Source: CAD feature listing. Evaluate the final solid. Frame: model axes, mm. A direction names the side the tool comes from. Give positions to 0.01 mm unless a question says otherwise; leave off trailing zeros. Order: outer loops, then holes, each group sorted by start corner. A loop starts at its lowest first (then second) coordinate and runs counter-clockwise, first axis right, second up.
```python
from build123d import *

# Parameters (mm, degrees)
F1_DEPTH  = 530
F0_R      = 50
F0_R_2    = 45
F2_DEPTH  = 9
F3_R      = 150.0861563529
F3_R_2    = 146
F3_R_3    = 144
F3_R_4    = 138
F4_DEPTH  = 15
F5_DEPTH  = 15
F7_R      = 141.9845884843
F8_DEPTH  = 15
F9_W      = 99.9695800245
F9_H      = 293.9526891708
F9_H_2    = 15
F10_DEPTH = 15
F11_W     = 99.9695800245
F11_H     = 308.8312447071
F12_DEPTH = 15
F14_DEPTH = 309
F15_DEPTH = 15
F16_DEPTH = 5
F17_R     = 2


with BuildPart() as f1:
    # F0 (on Front) → F1 (new body)
    with BuildSketch(Plane.XZ):
        with BuildLine():
            Line((50, 135.0407345952), (50, 137.1714255959))
            ThreePointArc((50, 137.1714255959), (0.000857941, 145.9999999975), (-49.9983878734, 137.1720132172))
            Line((-49.9983878734, 137.1720132172), (-49.9983878734, 135.041331488))
            ThreePointArc((-49.9983878734, 135.041331488), (0.0008595396, 143.9999999974), (50, 135.0407345952))
        make_face()
        with BuildLine():
            Line((-49.9983878734, 135.041331488), (-49.9983878734, 137.1720132172))
            ThreePointArc((-49.9983878734, 137.1720132172), (-146, 0), (-49.9983878734, -137.1720132172))
            Line((-49.9983878734, -137.1720132172), (-49.9983878734, -135.041331488))
            ThreePointArc((-49.9983878734, -135.041331488), (-144, 0), (-49.9983878734, 135.041331488))
        make_face()
        with BuildLine():
            ThreePointArc((-49.9983878734, -137.1720132172), (0.000857941, -145.9999999975), (50, -137.1714255959))
            Line((50, -137.1714255959), (50, -135.0407345952))
            ThreePointArc((50, -135.0407345952), (0.0008595396, -143.9999999974), (-49.9983878734, -135.041331488))
            Line((-49.9983878734, -135.041331488), (-49.9983878734, -137.1720132172))
        make_face()
        with BuildLine():
            ThreePointArc((146, 0), (119.6160524344, 83.7137981458), (50, 137.1714255959))
            Line((50, 137.1714255959), (50, 135.0407345952))
            ThreePointArc((50, 135.0407345952), (118.1862936216, 82.2678552048), (144, 0))
            ThreePointArc((144, 0), (118.1862936216, -82.2678552048), (50, -135.0407345952))
            Line((50, -135.0407345952), (50, -137.1714255959))
            ThreePointArc((50, -137.1714255959), (119.6160524344, -83.7137981458), (146, 0))
        make_face()
    extrude(amount=F1_DEPTH)

    # F0 (on Front) → F2 (join)
    with BuildSketch(Plane.XZ):
        with BuildLine():
            ThreePointArc((144, 0), (118.1862936216, 82.2678552048), (50, 135.0407345952))
            ThreePointArc((50, 135.0407345952), (0.0008595396, 143.9999999974), (-49.9983878734, 135.041331488))
            ThreePointArc((-49.9983878734, 135.041331488), (-144, 0), (-49.9983878734, -135.041331488))
            ThreePointArc((-49.9983878734, -135.041331488), (0.0008595396, -143.9999999974), (50, -135.0407345952))
            ThreePointArc((50, -135.0407345952), (118.1862936216, -82.2678552048), (144, 0))
        make_face()
        with BuildLine():
            Line((-59.3256604671, 60), (59.3256604671, 60))
            ThreePointArc((59.3256604671, 60), (62.8611943731, 58.5355339059), (64.3256604671, 55))
            Line((64.3256604671, 55), (64.3256604671, -55))
            ThreePointArc((64.3256604671, -55), (62.8611943731, -58.5355339059), (59.3256604671, -60))
            Line((59.3256604671, -60), (-59.3256604671, -60))
            ThreePointArc((-59.3256604671, -60), (-62.8611943731, -58.5355339059), (-64.3256604671, -55))
            Line((-64.3256604671, -55), (-64.3256604671, 55))
            ThreePointArc((-64.3256604671, 55), (-62.8611943731, 58.5355339059), (-59.3256604671, 60))
        make_face(mode=Mode.SUBTRACT)
        with BuildLine():
            Line((50, 137.1714255959), (50, 141.4213562373))
            ThreePointArc((50, 141.4213562373), (0.0008549575, 149.9999999976), (-49.9983878734, 141.4219261998))
            Line((-49.9983878734, 141.4219261998), (-49.9983878734, 137.1720132172))
            ThreePointArc((-49.9983878734, 137.1720132172), (0.000857941, 145.9999999975), (50, 137.1714255959))
        make_face()
        with BuildLine():
            Line((-49.9983878734, 137.1720132172), (-49.9983878734, 141.4219261998))
            ThreePointArc((-49.9983878734, 141.4219261998), (-150, 0), (-49.9983878734, -141.4219261998))
            Line((-49.9983878734, -141.4219261998), (-49.9983878734, -137.1720132172))
            ThreePointArc((-49.9983878734, -137.1720132172), (-146, 0), (-49.9983878734, 137.1720132172))
        make_face()
        with BuildLine():
            ThreePointArc((-49.9983878734, -141.4219261998), (0.0008549575, -149.9999999976), (50, -141.4213562373))
            Line((50, -141.4213562373), (50, -137.1714255959))
            ThreePointArc((50, -137.1714255959), (0.000857941, -145.9999999975), (-49.9983878734, -137.1720132172))
            Line((-49.9983878734, -137.1720132172), (-49.9983878734, -141.4219261998))
        make_face()
        with BuildLine():
            ThreePointArc((50, -141.4213562373), (122.4744871392, -86.6025403784), (150, 0))
            ThreePointArc((150, 0), (122.4744871392, 86.6025403784), (50, 141.4213562373))
            Line((50, 141.4213562373), (50, 137.1714255959))
            ThreePointArc((50, 137.1714255959), (119.6160524344, 83.7137981458), (146, 0))
            ThreePointArc((146, 0), (119.6160524344, -83.7137981458), (50, -137.1714255959))
            Line((50, -137.1714255959), (50, -141.4213562373))
        make_face()
        with BuildLine():
            ThreePointArc((64.3256604671, 55), (62.8611943731, 58.5355339059), (59.3256604671, 60))
            Line((59.3256604671, 60), (-59.3256604671, 60))
            ThreePointArc((-59.3256604671, 60), (-62.8611943731, 58.5355339059), (-64.3256604671, 55))
            Line((-64.3256604671, 55), (-64.3256604671, -55))
            ThreePointArc((-64.3256604671, -55), (-62.8611943731, -58.5355339059), (-59.3256604671, -60))
            Line((-59.3256604671, -60), (59.3256604671, -60))
            ThreePointArc((59.3256604671, -60), (62.8611943731, -58.5355339059), (64.3256604671, -55))
            Line((64.3256604671, -55), (64.3256604671, 55))
        make_face()
        Circle(F0_R, mode=Mode.SUBTRACT)
        Circle(F0_R)
        Circle(F0_R_2, mode=Mode.SUBTRACT)
    extrude(amount=F2_DEPTH)

    # F3 (on face) → F4 (join)
    with BuildSketch(Plane.XZ.offset(530)):
        Circle(F3_R)
        Circle(F3_R_2, mode=Mode.SUBTRACT)
        Circle(F3_R_2)
        Circle(F3_R_3, mode=Mode.SUBTRACT)
        Circle(F3_R_3)
        Circle(F3_R_4, mode=Mode.SUBTRACT)
    extrude(amount=-F4_DEPTH)

    # F0 (on Front) → F5 (join)
    with BuildSketch(Plane.XZ):
        with BuildLine():
            ThreePointArc((-49.9983878734, 141.4219261998), (0.0008549575, 149.9999999976), (50, 141.4213562373))
            Line((50, 141.4213562373), (50, 158))
            Line((50, 158), (-49.9983878734, 158))
            Line((-49.9983878734, 158), (-49.9983878734, 141.4219261998))
        make_face()
        with BuildLine():
            Line((50, -158), (50, -141.4213562373))
            ThreePointArc((50, -141.4213562373), (0.0008549575, -149.9999999976), (-49.9983878734, -141.4219261998))
            Line((-49.9983878734, -141.4219261998), (-49.9983878734, -158))
            Line((-49.9983878734, -158), (-34.5, -158))
            Line((-34.5, -158), (34.5, -158))
            Line((34.5, -158), (50, -158))
        make_face()
    extrude(amount=F5_DEPTH)

    # F7 (on offset) → F8 (join)
    with BuildSketch(Plane.XZ.offset(310)):
        Polygon((-91, 157.6166234888), (-182, 0), (-91, -157.6166234888), (91, -157.6166234888), (182, 0), (91, 157.6166234888), align=None)
        Circle(F7_R, mode=Mode.SUBTRACT)
    extrude(amount=-F8_DEPTH)

    # F9 (on face) → F10 (join)
    with BuildSketch(Plane.XY.offset(158)):
        with Locations((0.0152099878, -161.9763445854)):
            Rectangle(F9_W, F9_H)
        with Locations((0.0152099878, -7.5)):
            Rectangle(F9_W, F9_H_2)
    extrude(amount=F10_DEPTH)

    # F11 (on face) → F12 (join)
    with BuildSketch(Plane(origin=(0, 0, -158), x_dir=(1, 0, 0), z_dir=(0, 0, -1))):
        with Locations((0.0152099878, 154.4156223536)):
            Rectangle(F11_W, F11_H)
    extrude(amount=F12_DEPTH)

    # F13 (on face) → F14 (join)
    with BuildSketch(Plane.XZ.offset(308.8312447071)):
        Polygon((37, -179), (34.5, -173), (-34.5, -173), (-37, -179), align=None)
    extrude(amount=-F14_DEPTH)

    # F0 (on Front) → F15 (join)
    with BuildSketch(Plane.XZ):
        Circle(F0_R)
        Circle(F0_R_2, mode=Mode.SUBTRACT)
    extrude(amount=-F15_DEPTH)

    # F0 (on Front) → F16 (join)
    with BuildSketch(Plane.XZ):
        with BuildLine():
            ThreePointArc((64.3256604671, 55), (62.8611943731, 58.5355339059), (59.3256604671, 60))
            Line((59.3256604671, 60), (-59.3256604671, 60))
            ThreePointArc((-59.3256604671, 60), (-62.8611943731, 58.5355339059), (-64.3256604671, 55))
            Line((-64.3256604671, 55), (-64.3256604671, -55))
            ThreePointArc((-64.3256604671, -55), (-62.8611943731, -58.5355339059), (-59.3256604671, -60))
            Line((-59.3256604671, -60), (59.3256604671, -60))
            ThreePointArc((59.3256604671, -60), (62.8611943731, -58.5355339059), (64.3256604671, -55))
            Line((64.3256604671, -55), (64.3256604671, 55))
        make_face()
        Circle(F0_R, mode=Mode.SUBTRACT)
    extrude(amount=-F16_DEPTH)

    # F17
    f17_edges = [f1.edges().sort_by_distance(p)[0] for p in [
        (64.32566, 5, 0),
        (0, 5, 60),
        (-64.32566, 5, 0),
        (0, 5, -60),
        (-50, 5, 0),
    ]]
    fillet(f17_edges, radius=F17_R)


solid = f1.part
```
1) Pin query (flat end, axial travel): pin 1 (6 mm diameter, centred on x = 75.5, y = -435.5, fed in from -Z); pin 2 (1.5 mm diameter, centred on x = -101, y = -472.5, fed in from +Z); pin 3 (18 mm diameter, centred on x = 18.5, z = -152.5, fed in from -Y); pin 4 (2 mm diameter, centred on x = 93.5, z = 91.5, fed in from -Y). Return the tip coordinate at first contact, or that it passes through.
Report:
pin 1: stops at z = -126.73
pin 2: stops at z = 106.14
pin 3: stops at y = -530
pin 4: stops at y = -9
2) Draft query along X for faces 5 (the cylindrical face through (131.627, -522.605, 41.451)), 6 (the flat face through (135.863, -302.605, -79.912)), 7 (the flat face through (-41, 15, 19)). Return one class per face: +X half, -X half, draft (parallel to the pull), parting line (faces both ways), or undercut.
Report:
face 5: undercut
face 6: +X half
face 7: draft
3) Section query B-B, the plane y = -490. Return the cut outline in (x, z), and give its area (3 significant figures).
Report:
outline: circle Ø292 at (0, 0); hole circle Ø288 at (0, 0)
area: 1,820 mm2
4) Material intervals for L1, parallel to Z at x = 0, y = -100; L2, parallel to Y at x = -120.5, z = -78.5; L3, parallel to Z at x = 23, y = -9.5, sorted ascending.
Report:
L1: z = -179 to -158, -146 to -144, 144 to 146, 158 to 173
L2: y = -530 to -515, -310 to -295, -9 to 0
L3: z = -179 to -148.23, -144.18 to -142.15, 142.15 to 144.18, 148.23 to 173
5) Reachability of faces 1 (the flat face through (117, -515, -74)), 2 (the flat face through (-0.9, 5, 52.4)), 3 (the flat face through (-1, -152, 173)), 4 (the flat face through (-49.998, -7, -150)) from +Z, -Z, +X, -X, +Y, -Y: full face, straight path, thin tool, end or side. Return the list, or none.
Report:
face 1: none
face 2: +Y
face 3: +Z, +X, -X, +Y, -Y
face 4: -Z, -X, +Y
6) Section query A-A, the plane y = -211. Return the cut outline in (x, z).
Report:
outline: circle Ø292 at (0, 0); (-49.97, -173) - (-34.5, -173) - (-37, -179) - (37, -179) - (34.5, -173) - (50, -173) - (50, -158) - (-49.97, -158) - close; (-49.97, 158) - (50, 158) - (50, 173) - (-49.97, 173) - close; hole circle Ø288 at (0, 0)
